For this review, take the finished solid that the model builds, in its own axes (mm). Face numbers are marked on the shaded views. A direction names the side the tool comes from. Round coordinates to 2 decimals unless told otherwise and drop trailing zeros. Write each loop counter-clockwise with the first axis right and the second up, starting at its lowest first coordinate (ties: lowest second). Pieces come first, ordered by that corner, then holes. Notation, with made-up numbers: M -4,69.5 L 9,69.5 A13 ccw 9,92.5 Z; hole C 83.25,87.25 d11. An arc over 180 degrees is marked long. Answer in a Markdown table with one row per item.
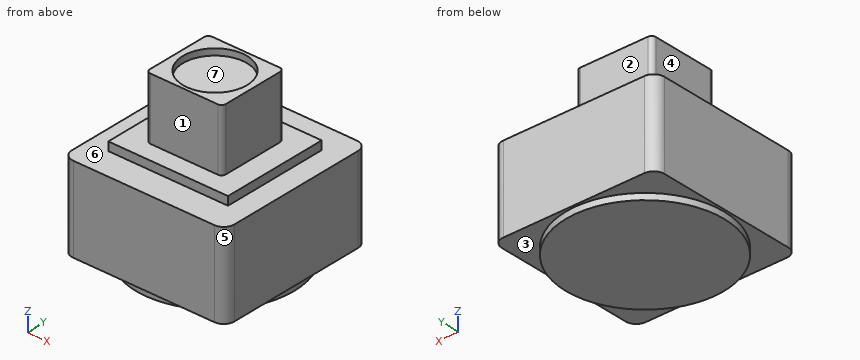
```python
from build123d import *

# Parameters (mm, degrees)
SKETCH1_W           = 96.52
SKETCH1_H           = 96.52
BOSS_EXTRUDE1_DEPTH = 50.8
SKETCH2_W           = 71.12
SKETCH2_H           = 63.5
BOSS_EXTRUDE2_DEPTH = 5.08
SKETCH3_W           = 45.212
SKETCH3_H           = 41.91
BOSS_EXTRUDE3_DEPTH = 36.83
SKETCH4_R           = 19.05
CUT_EXTRUDE1_DEPTH  = 3.81
SKETCH5_R           = 46.99
BOSS_EXTRUDE4_DEPTH = 3.81
FILLET1_R           = 2.54
FILLET2_R           = 6.35


with BuildPart() as part:
    # Sketch1 → Boss-Extrude1 (new body)
    with BuildSketch(Plane.XY):
        Rectangle(SKETCH1_W, SKETCH1_H)
    extrude(amount=BOSS_EXTRUDE1_DEPTH)

    # Sketch2 → Boss-Extrude2 (add)
    with BuildSketch(Plane.XY.offset(50.8)):
        Rectangle(SKETCH2_W, SKETCH2_H)
    extrude(amount=BOSS_EXTRUDE2_DEPTH)

    # Sketch3 → Boss-Extrude3 (add)
    with BuildSketch(Plane.XY.offset(55.88)):
        Rectangle(SKETCH3_W, SKETCH3_H)
    extrude(amount=BOSS_EXTRUDE3_DEPTH)

    # Sketch4 → Cut-Extrude1 (cut)
    with BuildSketch(Plane.XY.offset(92.71)):
        Circle(SKETCH4_R)
    extrude(amount=-CUT_EXTRUDE1_DEPTH, mode=Mode.SUBTRACT)

    # Sketch5 → Boss-Extrude4 (add)
    with BuildSketch(Plane(origin=(0, 0, 0), x_dir=(-1, 0, 0), z_dir=(0, 0, -1))):
        with Locations(Location((0, 0, 0), (0, 0, 180))):
            Circle(SKETCH5_R)
    extrude(amount=BOSS_EXTRUDE4_DEPTH)

    # Fillet1
    fillet1_edges = [part.edges().sort_by_distance(p)[0] for p in [
        (22.606, -20.955, 74.295),
        (22.606, 20.955, 74.295),
        (-22.606, 20.955, 74.295),
        (-22.606, -20.955, 74.295),
    ]]
    fillet(fillet1_edges, radius=FILLET1_R)

    # Fillet2
    fillet2_edges = [part.edges().sort_by_distance(p)[0] for p in [
        (48.26, -48.26, 25.4),
        (-48.26, -48.26, 25.4),
        (-48.26, 48.26, 25.4),
        (48.26, 48.26, 25.4),
    ]]
    fillet(fillet2_edges, radius=FILLET2_R)


solid = part.part
```
Q1. Machinability: for the marked faces 1, 2, 3 and 4, which of the approach directions +Z, -Z, +X, -X, +Y, -Y give a long, thin tool a straight path to every point of the face, cutting with its end or side? Answer none if there is none.
Found:
| item | result |
|---|---|
| face 1 | +Z, +X, -X, -Y |
| face 2 | +Z, +X, -X, +Y |
| face 3 | -Z |
| face 4 | +Z, -X, +Y, -Y |
Q2. Take a section at D-D (x = -30). State the section outline as (y, z) points, then the cut area to 3 significant figures.
Found:
| item | result |
|---|---|
| outline | M -48.26,0 L -36.17,0 L -36.17,-3.81 L 36.17,-3.81 L 36.17,0 L 48.26,0 L 48.26,50.8 L 31.75,50.8 L 31.75,55.88 L -31.75,55.88 L -31.75,50.8 L -48.26,50.8 Z |
| area | 5,500 mm² |
Q3. Take a section at B-B (y = 0). State the section outline as (x, z) points.
Found:
| item | result |
|---|---|
| outline | M -48.26,0 L -46.99,0 L -46.99,-3.81 L 46.99,-3.81 L 46.99,0 L 48.26,0 L 48.26,50.8 L 35.56,50.8 L 35.56,55.88 L 22.61,55.88 L 22.61,92.71 L 19.05,92.71 L 19.05,88.9 L -19.05,88.9 L -19.05,92.71 L -22.61,92.71 L -22.61,55.88 L -35.56,55.88 L -35.56,50.8 L -48.26,50.8 Z |
Q4. Mouldability with a two-part tool opening along Y and no side actions: class the marked faces 5, 6 and 7 as +Y half, -Y half, draft (parallel to the pull), parting line (faces both ways), or undercut.
Found:
| item | result |
|---|---|
| face 5 | -Y half |
| face 6 | draft |
| face 7 | undercut |
Q5. Take a section at C-C (x = 0). State the section outline as (y, z) points (3 decimals), then the cut area to 3 significant figures.
Found:
| item | result |
|---|---|
| outline | M -48.26,0 L -46.99,0 L -46.99,-3.81 L 46.99,-3.81 L 46.99,0 L 48.26,0 L 48.26,50.8 L 31.75,50.8 L 31.75,55.88 L 20.955,55.88 L 20.955,92.71 L 19.05,92.71 L 19.05,88.9 L -19.05,88.9 L -19.05,92.71 L -20.955,92.71 L -20.955,55.88 L -31.75,55.88 L -31.75,50.8 L -48.26,50.8 Z |
| area | 6,980 mm² |
Q6. Insertion check: P1, Ø5.5, axis at x = 1.5, z = 54, coming from the +Y side; P2, Ø18.5, axis at x = 2.5, z = 80.5, coming from the +Y side (3 decimals); P3, Ø5.5, axis at x = 15, z = 53, coming from the -Y side; P4, Ø3, axis at x = 27.5, y = 12.5, coming from the +Z side. Each pin has a flat end and moves straight along its axis. Give the tip position at first contact, or say it passes through.
Found:
| item | result |
|---|---|
| P1 | y = 31.75 |
| P2 | y = 20.955 |
| P3 | y = -48.26 |
| P4 | z = 55.88 |
Q7. For probe 1 along Y at (x, z) = (0, 90) (3 decimals); probe 2 along Z at (x, y) = (28, 36); probe 3 along Y at (x, z) = (-22, 65), list the stretches that pass through material, from the lowest coordinate up.
Found:
| item | result |
|---|---|
| probe 1 | -20.955 to -19.05, 19.05 to 20.955 |
| probe 2 | -3.81 to 50.8 |
| probe 3 | -20.06 to 20.06 |
Q8. Take a section at A-A (z = 57.5). State the section outline as (x, y) points (3 decimals), then the cut area to 3 significant figures.
Found:
| item | result |
|---|---|
| outline | M -22.606,-18.415 A2.54 ccw -20.066,-20.955 L 20.066,-20.955 A2.54 ccw 22.606,-18.415 L 22.606,18.415 A2.54 ccw 20.066,20.955 L -20.066,20.955 A2.54 ccw -22.606,18.415 Z |
| area | 1,890 mm² |
